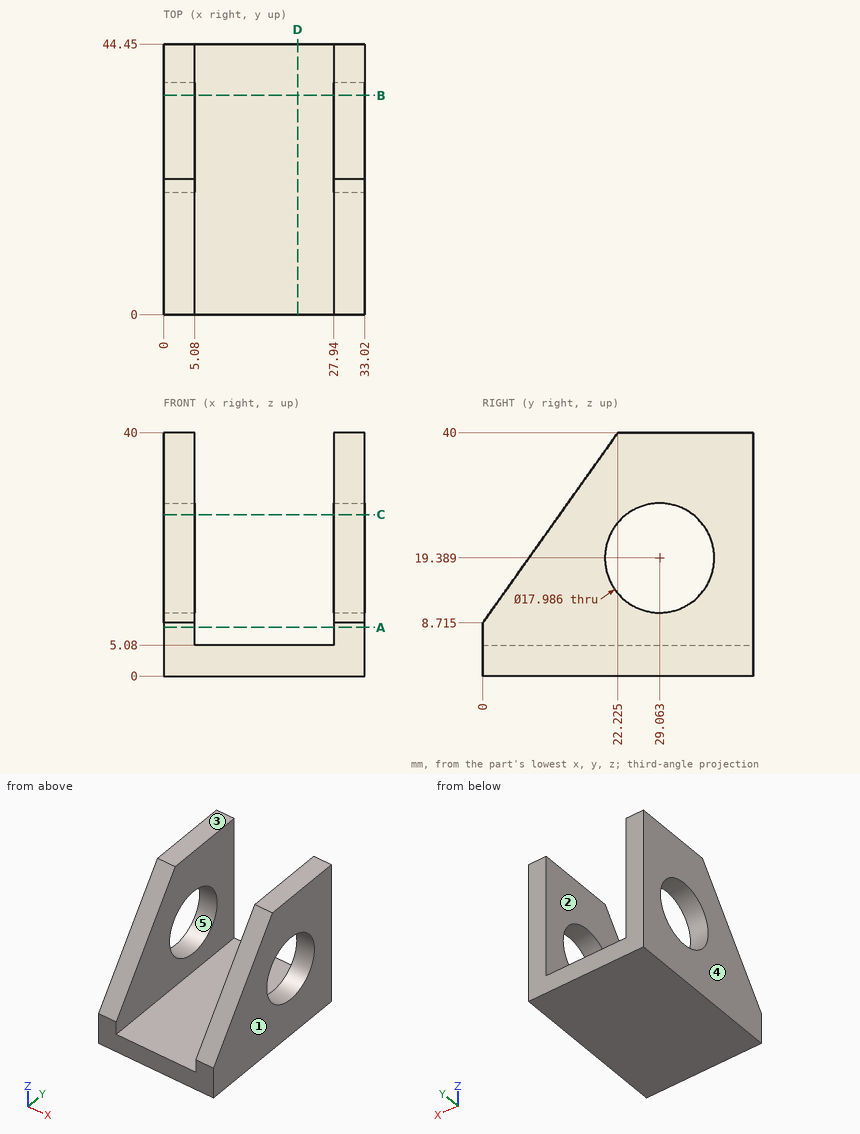
Input: dimensioned drawing with shaded views. Units: mm. Origin: part minimum x, y, z. A direction names the side the tool comes from. Coordinates: 2 decimals unless noted, no trailing zeros. Loops run counter-clockwise (first coordinate to the right, second up) from the corner with the lowest first, then second, coordinate; pieces in that order, holes last. Notation, with made-up numbers: (-5.5, -22.5) -> (22.5, -22.5) arc R12 ccw to (22.5, -15.5) -> close; hole circle Ø9 at (-8.75, 45.25). An arc over 180 degrees is marked (long way). One line per item, written item: value. Start each with the question number.
Q1. Section query D-D, the plane x = 22. Return the cut outline in (y, z), and give its area (3 significant figures).
Q2. Contact query for flat-ended pins moving along their axis: P1, Ø10, axis at x = 22.5, y = 29.5, coming from the +Z side; P2, Ø12, axis at x = 9, z = 28.5, coming from the -Y side. Output: stop coordinate, or through.
Q3. Mould query, pull axis Z, two halves, no side actions, for the marked faces 3, 4 and 5. Classes: pulls with the +Z half, pulls with the -Z half, needs draft (parallel to the pull), parting line crosses it, or undercut.
Q4. Section query B-B, the plane y = 36. Return the cut outline in (x, z), and give its area (3 significant figures).
Q5. Set-up query: the marked faces 1 and 2. Return all of +Z, -Z, +X, -X, +Y, -Y with unobstructed straight access to the full face (end or side cutting, diameter ignored); none if empty.
Q6. Section query A-A, the plane z = 8. Return the cut outline in (x, y).
Q7. Section query C-C, the plane z = 26.5. Give the number of separate pieces and of enclosed holes in the cut face, and give its area (3 significant figures).
Q8. Line query: line 1 along X through (y, z) = (23, 12); line 2 along Z through (x, y) = (6, 18); line 3 along Z through (x, y) = (31, 28.5) (1 decimal). Output: solid intervals per line, ascending.
Results:
1. outline: (0, 0) -> (44.45, 0) -> (44.45, 5.08) -> (0, 5.08) -> close
1. area: 226 mm^2
2. P1: z = 5.08
2. P2: y = 10.83
3. face 3: pulls with the +Z half
3. face 4: needs draft
3. face 5: undercut
4. outline: (0, 0) -> (33.02, 0) -> (33.02, 13.67) -> (27.94, 13.67) -> (27.94, 5.08) -> (5.08, 5.08) -> (5.08, 13.67) -> (0, 13.67) -> close; (0, 25.11) -> (5.08, 25.11) -> (5.08, 40) -> (0, 40) -> close; (27.94, 25.11) -> (33.02, 25.11) -> (33.02, 40) -> (27.94, 40) -> close
4. area: 406 mm^2
5. face 1: +Z, -Z, +X, +Y, -Y
5. face 2: +Z, +Y, -Y
6. outline: (0, 0) -> (5.08, 0) -> (5.08, 44.45) -> (0, 44.45) -> close; (27.94, 0) -> (33.02, 0) -> (33.02, 44.45) -> (27.94, 44.45) -> close
7. separate pieces: 4
7. enclosed holes: 0
7. area: 211 mm^2
8. line 1: 0 to 5.08, 27.94 to 33.02
8. line 2: 0 to 5.08
8. line 3: 0 to 10.4, 28.4 to 40
